Design review of the part built by this model. Coordinates are the model's own, in mm. Face numbers are marked on the shaded views. A direction names the side the tool comes from. Coordinates: 2 decimals unless noted, no trailing zeros. Loops run counter-clockwise (first coordinate to the right, second up) from the corner with the lowest first, then second, coordinate; pieces in that order, holes last. Notation, with made-up numbers: M 70.25,-13.75 L 86.25,-13.75 A11 ccw 86.25,7.25 Z; hole C -29,-28 d1. An arc over 180 degrees is marked long. Answer as CSV lines item,"result". Start each with the question number.
from build123d import *

# Parameters (mm, degrees)
F0_R     = 25.216468
F1_DEPTH = 35.56
F2_W     = 20.449843
F2_H     = 33.23099
F3_DEPTH = 28.956
F5_R     = 10.26144
F6_DEPTH = 65.532


with BuildPart() as f1:
    # F0 (on Top) → F1 (new body)
    with BuildSketch(Plane.XY):
        Circle(F0_R)
    extrude(amount=F1_DEPTH)

    # F2 (on Top) → F3 (cut)
    with BuildSketch(Plane.XY):
        with Locations((-0.383434, 0)):
            Rectangle(F2_W, F2_H)
    extrude(amount=F3_DEPTH, mode=Mode.SUBTRACT)

    # F5 (on offset) → F6 (cut)
    with BuildSketch(Plane.YZ.offset(30.226)):
        with Locations((0, 13.160355)):
            Circle(F5_R)
    extrude(amount=-F6_DEPTH, mode=Mode.SUBTRACT)


solid = f1.part
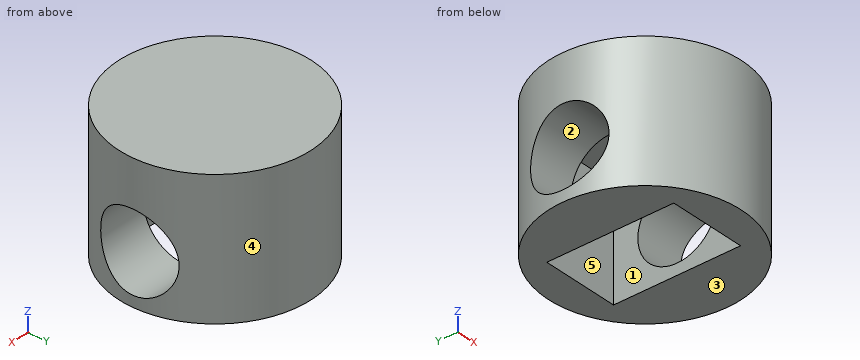
Item 1: Add section B-B (z = 9.5). Give the boundary of the cut face in (x, y), plus the area to 3 significant figures.
Item 2: Add section C-C (x = 0). Give the boundary of the cut face in (y, z).
Item 3: For pin 1 (5 mm diameter, centred on y = 16, z = 8, fed in from -X); pin 2 (2 mm diameter, centred on x = -10, z = 13, fed in from -Y); pin 3 (8 mm diameter, centred on y = 17.5, z = 16.5, fed in from +X); pin 4 (18.5 mm diameter, centred on y = 0, z = 13.16, fed in from -X), all flat-tipped, find the tip position at first contact; note any pin that passes through.
Item 4: Add section A-A (y = 0). Give the boundary of the cut face in (x, z).
Item 5: For line 1 along Z through (x, y) = (-20, 0); line 2 along Z through (x, y) = (-5, -8); line 3 along X through (y, z) = (0.5, 27), list the stretches that pass through material, from the lowest coordinate up. Write a range as from..to.
Item 6: Mouldability with a two-part tool opening along Z and no side actions: class the marked faces 1, 2 and 3 as released by +Z, released by -Z, zero draft, split by the parting line, or undercut.
Item 7: For the marked faces 4 and 5, list the 3-axis set-ups (+Z, -Z, +X, -X, +Y, -Y) from which the entire face can be reached by the end or side of a thin tool; tool diameter is ignored.
Item 8: Add section D-D (z = 27). Give the boundary of the cut face in (x, y), plus the area to 3 significant figures.
Response:
1,outline,"M -23.32,-9.59 A25.22 ccw 23.32,-9.59 L 9.84,-9.59 L 9.84,-16.62 L -10.61,-16.62 L -10.61,-9.59 Z; M -23.32,9.59 L -10.61,9.59 L -10.61,16.62 L 9.84,16.62 L 9.84,9.59 L 23.32,9.59 A25.22 ccw Z"
1,area,"767 mm²"
2,outline,"M -25.22,0 L -16.62,0 L -16.62,28.96 L 16.62,28.96 L 16.62,0 L 25.22,0 L 25.22,35.56 L -25.22,35.56 Z"
3,pin 1,"x = -21.3"
3,pin 2,"y = -23.56"
3,pin 3,"x = 21.3"
3,pin 4,"through"
4,outline,"M -25.22,0 L -10.61,0 L -10.61,2.9 L -25.22,2.9 Z; M -25.22,23.42 L -10.61,23.42 L -10.61,28.96 L 9.84,28.96 L 9.84,23.42 L 25.22,23.42 L 25.22,35.56 L -25.22,35.56 Z; M 9.84,0 L 25.22,0 L 25.22,2.9 L 9.84,2.9 Z"
5,line 1,"0..2.9, 23.42..35.56"
5,line 2,"28.96..35.56"
5,line 3,"-25.21..-10.61, 9.84..25.21"
6,face 1,"zero draft"
6,face 2,"undercut"
6,face 3,"released by -Z"
7,face 4,"+Z, -Z"
7,face 5,"-Z"
8,outline,"C 0,0 d50.43; hole M -10.61,-16.62 L 9.84,-16.62 L 9.84,16.62 L -10.61,16.62 Z"
8,area,"1,320 mm²"
